Geometry: final body of the model. Coordinates: model frame, mm. A direction names the side the tool comes from. Give positions to 0.01 mm unless a question says otherwise; leave off trailing zeros. Loops run counter-clockwise (first coordinate to the right, second up) from the corner with the lowest first, then second, coordinate; pieces in that order, holes last.
from build123d import *

# Parameters (mm, degrees)
EXTRUDE_1_DEPTH     = 76
SKETCH_2_R          = 19.05
EXTRUDE_2_DEPTH     = 1.6
SKETCH_3_OUTSIDE_W  = 80.656
SKETCH_3_OUTSIDE_H  = 80.656
CUT_EXTRUDE_1_DEPTH = 71.2
SKETCH_4_R          = 2.55
CUT_EXTRUDE_2_DEPTH = 71.2
SKETCH_5_R          = 3.175
EXTRUDE_3_DEPTH     = 19.4


with BuildPart() as part:
    # Эскиз1 → Бобышка-Вытянуть1 (new body)
    with BuildSketch(Plane.XY):
        with BuildLine():
            Line((5, 0), (51.4, 0))
            ThreePointArc((51.4, 0), (54.935533906, 1.464466094), (56.4, 5))
            Line((56.4, 5), (56.4, 51.4))
            ThreePointArc((56.4, 51.4), (54.935533906, 54.935533906), (51.4, 56.4))
            Line((51.4, 56.4), (5, 56.4))
            ThreePointArc((5, 56.4), (1.464466094, 54.935533906), (0, 51.4))
            Line((0, 51.4), (0, 5))
            ThreePointArc((0, 5), (1.464466094, 1.464466094), (5, 0))
        make_face()
    extrude(amount=EXTRUDE_1_DEPTH)

    # Эскиз2 → Бобышка-Вытянуть2 (add)
    with BuildSketch(Plane.XY.offset(76)):
        with Locations(Location((28.2, 28.2, 0), (0, 0, 180))):
            Circle(SKETCH_2_R)
    extrude(amount=EXTRUDE_2_DEPTH)

    # Эскиз3 outside → Вырез-Вытянуть1 (cut)
    with BuildSketch(Plane(origin=(0, 0, 0), x_dir=(-1, 0, 0), z_dir=(0, 0, -1))):
        with Locations((-28.2, 28.2)):
            Rectangle(SKETCH_3_OUTSIDE_W, SKETCH_3_OUTSIDE_H)
        with BuildLine():
            Line((-56.4, 11), (-56.4, 45.4))
            ThreePointArc((-56.4, 45.4), (-55.814213562, 46.814213562), (-54.4, 47.4))
            Line((-54.4, 47.4), (-49.4, 47.4))
            ThreePointArc((-49.4, 47.4), (-47.985786438, 47.985786438), (-47.4, 49.4))
            Line((-47.4, 49.4), (-47.4, 54.4))
            ThreePointArc((-47.4, 54.4), (-46.814213562, 55.814213562), (-45.4, 56.4))
            Line((-45.4, 56.4), (-11, 56.4))
            ThreePointArc((-11, 56.4), (-9.585786438, 55.814213562), (-9, 54.4))
            Line((-9, 54.4), (-9, 49.4))
            ThreePointArc((-9, 49.4), (-8.414213562, 47.985786438), (-7, 47.4))
            Line((-7, 47.4), (-2, 47.4))
            ThreePointArc((-2, 47.4), (-0.585786438, 46.814213562), (0, 45.4))
            Line((0, 45.4), (0, 11))
            ThreePointArc((0, 11), (-0.585786438, 9.585786438), (-2, 9))
            Line((-2, 9), (-7, 9))
            ThreePointArc((-7, 9), (-8.414213562, 8.414213562), (-9, 7))
            Line((-9, 7), (-9, 2))
            ThreePointArc((-9, 2), (-9.585786438, 0.585786438), (-11, 0))
            Line((-11, 0), (-45.4, 0))
            ThreePointArc((-45.4, 0), (-46.814213562, 0.585786438), (-47.4, 2))
            Line((-47.4, 2), (-47.4, 7))
            ThreePointArc((-47.4, 7), (-47.985786438, 8.414213562), (-49.4, 9))
            Line((-49.4, 9), (-54.4, 9))
            ThreePointArc((-54.4, 9), (-55.814213562, 9.585786438), (-56.4, 11))
        make_face(mode=Mode.SUBTRACT)
    extrude(amount=-CUT_EXTRUDE_1_DEPTH, mode=Mode.SUBTRACT)

    # Эскиз4 → Вырез-Вытянуть2 (cut)
    with BuildSketch(Plane.XY.offset(76)):
        with Locations((4.63, 51.77)):
            Circle(SKETCH_4_R)
        with Locations(Location((51.77, 51.77, 0), (0, 0, 180))):
            Circle(SKETCH_4_R)
        with Locations(Location((4.63, 4.63, 0), (0, 0, 180))):
            Circle(SKETCH_4_R)
        with Locations((51.77, 4.63)):
            Circle(SKETCH_4_R)
    extrude(amount=-CUT_EXTRUDE_2_DEPTH, mode=Mode.SUBTRACT)

    # Эскиз5 → Бобышка-Вытянуть3 (add)
    with BuildSketch(Plane.XY.offset(77.6)):
        with Locations((28.2, 28.2)):
            Circle(SKETCH_5_R)
    extrude(amount=EXTRUDE_3_DEPTH)


solid = part.part
Item 1: Section query B-B on z = 56.5. Return loops of the section in (x, y), plus the area to 3 significant figures.
Values follow:
outline: (0, 11) arc R2 ccw to (2, 9) - (7, 9) arc R2 cw to (9, 7) - (9, 2) arc R2 ccw to (11, 0) - (45.4, 0) arc R2 ccw to (47.4, 2) - (47.4, 7) arc R2 cw to (49.4, 9) - (54.4, 9) arc R2 ccw to (56.4, 11) - (56.4, 45.4) arc R2 ccw to (54.4, 47.4) - (49.4, 47.4) arc R2 cw to (47.4, 49.4) - (47.4, 54.4) arc R2 ccw to (45.4, 56.4) - (11, 56.4) arc R2 ccw to (9, 54.4) - (9, 49.4) arc R2 cw to (7, 47.4) - (2, 47.4) arc R2 ccw to (0, 45.4) - close
area: 2,850 mm2
Item 2: Ray query, probe 1 along Y at (x, z) = (51.77, 72.7); probe 2 along X at (y, z) = (4, 72); probe 3 along Z at (x, y) = (31, 25.5). Return the intervals inside material, ascending.
Values follow:
probe 1: y = 0.01 to 2.08, 7.18 to 49.22, 54.32 to 56.39
probe 2: x = 0.1 to 2.16, 7.1 to 49.3, 54.24 to 56.3
probe 3: z = 0 to 77.6
Item 3: Pin query (flat end, axial travel): pin 1 (6 mm diameter, centred on x = 44, y = 15, fed in from +Z); pin 2 (2.5 mm diameter, centred on y = 50.5, z = 42.5, fed in from -X); pin 3 (3 mm diameter, centred on x = 6.5, z = 36.5, fed in from -Y). Return the tip coordinate at first contact, or that it passes through.
Values follow:
pin 1: stops at z = 77.6
pin 2: stops at x = 8.99
pin 3: stops at y = 8.73
Item 4: Section query D-D on x = 18. Return loops of the section in (y, z).
Values follow:
outline: (0, 0) - (56.4, 0) - (56.4, 76) - (44.29, 76) - (44.29, 77.6) - (12.11, 77.6) - (12.11, 76) - (0, 76) - close
Item 5: Draft query along Y for faces 4 (the face through (29, 56.4, 37)), 5 (the face through (4, 9, 35)), 6 (the face through (9, 52, 35)), 7 (the face through (2.2, 3.86, 73.63)). Return one class per face: +Y half, -Y half, draft (parallel to the pull), parting line (faces both ways), or undercut.
Values follow:
face 4: +Y half
face 5: -Y half
face 6: draft
face 7: undercut
Item 6: Section query A-A on x = 28.2. Return loops of the section in (y, z) (3 decimals).
Values follow:
outline: (0, 0) - (56.4, 0) - (56.4, 76) - (47.25, 76) - (47.25, 77.6) - (31.375, 77.6) - (31.375, 97) - (25.025, 97) - (25.025, 77.6) - (9.15, 77.6) - (9.15, 76) - (0, 76) - close
Item 7: Set-up query: faces 1 (the face through (8.43, 48, 35.1)), 2 (the face through (55.8, 9.57, 35.1)), 3 (the face through (27.51, 25.1, 87.16)). Return all of +Z, -Z, +X, -X, +Y, -Y with unobstructed straight access to the full face (end or side cutting, diameter ignored); none if empty.
Values follow:
face 1: -Z, -X, +Y
face 2: -Z, +X, -Y
face 3: +Z
